```python
from build123d import *

# Parameters (mm, degrees)
SKETCH1_W                 = 31.75
SKETCH1_H                 = 31.75
BOSS_EXTRUDE1_DEPTH       = 5.08
M3_CLEARANCE_HOLE1_D      = 3.4
M3_CLEARANCE_HOLE1_DEPTH  = 15.24
M3_CLEARANCE_HOLE1_TIP    = 1.021463052
SKETCH7_W                 = 31.75
SKETCH7_H                 = 31.75
SKETCH7_R                 = 13.97
BOSS_EXTRUDE2_DEPTH       = 24
M3X0_5_TAPPED_HOLE1_D     = 2.5
M3X0_5_TAPPED_HOLE1_DEPTH = 15.24
M3X0_5_TAPPED_HOLE1_TIP   = 0.751075774
SKETCH12_R                = 4.7625
CUT_EXTRUDE1_DEPTH        = 6.35
CUT_EXTRUDE2_REACH        = 44.849
CUT_EXTRUDE2_END_RADIUS   = 13.97
SKETCH13_W                = 15.618932536
SKETCH13_H                = 11.098734185
CIRPATTERN1_COUNT         = 4
CIRPATTERN2_COUNT         = 4


with BuildPart() as part:
    # Sketch1 → Boss-Extrude1 (new body)
    with BuildSketch(Plane(origin=(0, 0, 0), x_dir=(1, 0, 0), z_dir=(0, 1, 0))):
        Rectangle(SKETCH1_W, SKETCH1_H)
    extrude(amount=BOSS_EXTRUDE1_DEPTH)

    # M3 Clearance Hole1
    with Locations(Plane(origin=(0, 5.08, 0), x_dir=(1, 0, 0), z_dir=(0, 1, 0))):
        with Locations((-5.656854249, 5.656854249), (6.717514421, 6.717514421), (5.656854249, -5.656854249), (-6.717514421, -6.717514421)):
            Hole(M3_CLEARANCE_HOLE1_D / 2, depth=M3_CLEARANCE_HOLE1_DEPTH)
            with Locations((0, 0, -(M3_CLEARANCE_HOLE1_DEPTH + M3_CLEARANCE_HOLE1_TIP / 2))):  # 118° drill point
                Cone(0, M3_CLEARANCE_HOLE1_D / 2, M3_CLEARANCE_HOLE1_TIP, mode=Mode.SUBTRACT)

    # Sketch7 → Boss-Extrude2 (add)
    with BuildSketch(Plane.XZ):
        Rectangle(SKETCH7_W, SKETCH7_H)
        with Locations(Location((0, 0, 0), (0, 0, 270))):
            Circle(SKETCH7_R, mode=Mode.SUBTRACT)
    extrude(amount=BOSS_EXTRUDE2_DEPTH)

    # M3x0.5 Tapped Hole1
    with Locations(Plane(origin=(0, -24, 0), x_dir=(-1, 0, 0), z_dir=(0, -1, 0))):
        with Locations((-12.7, 12.7), (12.7, 12.7), (12.7, -12.7), (-12.7, -12.7)):
            Hole(M3X0_5_TAPPED_HOLE1_D / 2, depth=M3X0_5_TAPPED_HOLE1_DEPTH)
            with Locations((0, 0, -(M3X0_5_TAPPED_HOLE1_DEPTH + M3X0_5_TAPPED_HOLE1_TIP / 2))):  # 118° drill point
                Cone(0, M3X0_5_TAPPED_HOLE1_D / 2, M3X0_5_TAPPED_HOLE1_TIP, mode=Mode.SUBTRACT)

    # Sketch12 → Cut-Extrude1 (cut)
    with BuildSketch(Plane(origin=(0, 0, -15.875), x_dir=(-1, 0, 0), z_dir=(0, 0, -1))):
        with Locations((0, -1.27)):
            Circle(SKETCH12_R)
    cut_extrude1 = extrude(amount=-CUT_EXTRUDE1_DEPTH, mode=Mode.SUBTRACT)

    # Cut-Extrude2: up to this cylinder (the profile starts outside it)
    cut_extrude2_end = Plane(origin=(0, -14.261548, 0), z_dir=(0, 1, 0)) * Cylinder(CUT_EXTRUDE2_END_RADIUS, 118.638, mode=Mode.PRIVATE)
    # Sketch13 → Cut-Extrude2 (cut, up to the surface)
    with BuildSketch(Plane(origin=(0, 0, -15.875), x_dir=(-1, 0, 0), z_dir=(0, 0, -1)), mode=Mode.PRIVATE) as cut_extrude2_sk1:
        with Locations((0, -14.261548471)):
            Rectangle(SKETCH13_W, SKETCH13_H)
    cut_extrude2_tool1 = extrude(cut_extrude2_sk1.sketch, amount=-CUT_EXTRUDE2_REACH, mode=Mode.PRIVATE) - cut_extrude2_end
    cut_extrude2 = cut_extrude2_tool1.solids().sort_by_distance((0, -14.261548, -15.875))[0]
    add(cut_extrude2, mode=Mode.SUBTRACT)

    # CirPattern1: Cut-Extrude2 ×4 about axis
    cirpattern1_axis = Axis((0, 0, 0), (0, 1, 0))
    for i in range(1, CIRPATTERN1_COUNT):
        add(cut_extrude2.rotate(cirpattern1_axis, i * 360 / CIRPATTERN1_COUNT), mode=Mode.SUBTRACT)

    # CirPattern2: Cut-Extrude1 ×4 about axis
    cirpattern2_axis = Axis((0, 0, 0), (0, 1, 0))
    for i in range(1, CIRPATTERN2_COUNT):
        add(cut_extrude1.rotate(cirpattern2_axis, i * 360 / CIRPATTERN2_COUNT), mode=Mode.SUBTRACT)


solid = part.part
```
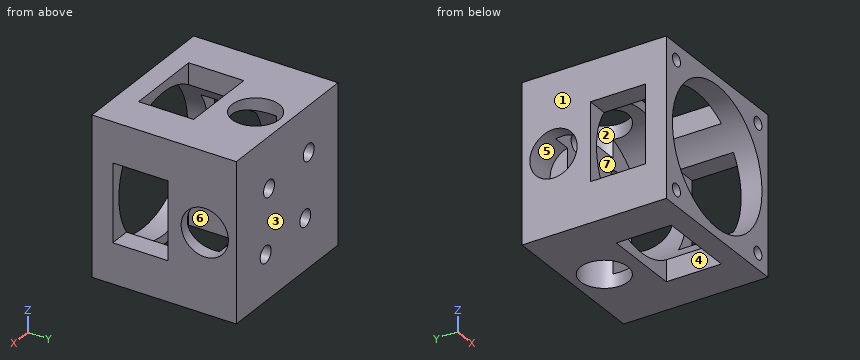
Work out the finished part from the listing and answer in its coordinate system (mm). Face numbers are marked on the shaded views. A direction names the side the tool comes from. Give positions to 0.01 mm unless a question says otherwise; leave off trailing zeros. Loops run counter-clockwise (first coordinate to the right, second up) from the corner with the lowest first, then second, coordinate; pieces in that order, holes last. Notation, with made-up numbers: (76, 37) -> (80, 37) arc R23 ccw to (80, 48) -> close; hole circle Ø11 at (46.5, 4). An arc over 180 degrees is marked (long way). Use CSV: the item, a comma, the result in double quotes.
1. The part is cut by section B-B (x = -1). Write down the section's boundary in (y, z) (3 decimals).
Found:
outline,"(-24, -15.875) -> (-19.811, -15.875) -> (-19.811, -13.934) -> (-24, -13.934) -> close; (-24, 13.934) -> (-19.811, 13.934) -> (-19.811, 15.875) -> (-24, 15.875) -> close; (-8.712, -15.875) -> (-5.926, -15.875) -> (-5.926, -13.934) -> (-8.712, -13.934) -> close; (-8.712, 13.934) -> (-5.926, 13.934) -> (-5.926, 15.875) -> (-8.712, 15.875) -> close; (0, -9.525) -> (3.386, -9.525) -> (3.386, -15.875) -> (5.08, -15.875) -> (5.08, 15.875) -> (3.386, 15.875) -> (3.386, 9.525) -> (0, 9.525) -> close"
2. The part is cut by section A-A (y = -14.5). Write down the section's boundary in (x, z) (3 decimals).
Found:
outline,"(-15.875, -15.875) -> (-7.809, -15.875) -> (-7.809, -11.583) arc R13.97 cw to (-11.583, -7.809) -> (-15.875, -7.809) -> close; (-15.875, 7.809) -> (-11.583, 7.809) arc R13.97 cw to (-7.809, 11.583) -> (-7.809, 15.875) -> (-15.875, 15.875) -> close; (7.809, -15.875) -> (15.875, -15.875) -> (15.875, -7.809) -> (11.583, -7.809) arc R13.97 cw to (7.809, -11.583) -> close; (7.809, 11.583) arc R13.97 cw to (11.583, 7.809) -> (15.875, 7.809) -> (15.875, 15.875) -> (7.809, 15.875) -> close; hole circle Ø2.5 at (-12.7, -12.7); hole circle Ø2.5 at (-12.7, 12.7); hole circle Ø2.5 at (12.7, -12.7); hole circle Ø2.5 at (12.7, 12.7)"
3. A tool of negligible diameter and unlimited length cuts with its end or side. For the marked faces 5, 6 and 7, from which of +Z, -Z, +X, -X, +Y, -Y can it reach the whole face along a straight path? Write none if from no direction.
Found:
face 5,"-X"
face 6,"+Z, -Z"
face 7,"-Y"
4. Straight lines are drawn through the part: line 1 (X direction, y = -17.75, z = -12.7) (3 decimals); line 2 (X direction, y = 1, z = -6.5) (3 decimals). For each, find the intervals that lie inside material, in ascending order.
Found:
line 1,"-15.875 to -13.95, -11.45 to -7.809, 7.809 to 11.45, 13.95 to 15.875"
line 2,"-15.875 to -7.133, -4.181 to 5.031, 8.404 to 15.875"
5. The mould has two halves that part along Y. Classify the marked faces 1, 2, 3 and 4: +Y half, -Y half, draft (parallel to the pull), parting line (faces both ways), or undercut.
Found:
face 1,"draft"
face 2,"undercut"
face 3,"+Y half"
face 4,"undercut"
6. Flat-ended cylindrical pins translate along their axes: pin 1 Ø8 at (x, z) = (-0.5, -4) entering from -Y; pin 2 Ø1.5 at (x, y) = (-3, -1) entering from -Z; pin 3 Ø1.5 at (x, z) = (-12.7, -12.7) entering from -Y; pin 4 Ø1.7 at (x, y) = (0, 1) entering from +Z (3 decimals). Find the tip coordinate at first contact, or state that the pin passes through.
Found:
pin 1,"y = 0"
pin 2,"through"
pin 3,"y = -8.46"
pin 4,"z = 9.525"
7. The part is cut by section D-D (z = -2). Write down the section's boundary in (x, y) (3 decimals), then the cut area to 3 significant figures.
Found:
outline,"(-15.875, -24) -> (-13.826, -24) -> (-13.826, -19.811) -> (-15.875, -19.811) -> close; (-15.875, -8.712) -> (-13.826, -8.712) -> (-13.826, -5.592) -> (-15.875, -5.592) -> close; (-15.875, 3.052) -> (-9.525, 3.052) -> (-9.525, 0) -> (9.525, 0) -> (9.525, 3.052) -> (15.875, 3.052) -> (15.875, 5.08) -> (-15.875, 5.08) -> close; (13.826, -24) -> (15.875, -24) -> (15.875, -19.811) -> (13.826, -19.811) -> close; (13.826, -8.712) -> (15.875, -8.712) -> (15.875, -5.592) -> (13.826, -5.592) -> close"
area,"152 mm^2"
8. The part is cut by section C-C (y = 3). Write down the section's boundary in (x, z) (3 decimals), then the cut area to 3 significant figures.
Found:
outline,"(-15.875, -15.875) -> (-2.109, -15.875) -> (-2.109, -9.525) -> (2.109, -9.525) -> (2.109, -15.875) -> (15.875, -15.875) -> (15.875, -2.109) -> (9.525, -2.109) -> (9.525, 2.109) -> (15.875, 2.109) -> (15.875, 15.875) -> (2.109, 15.875) -> (2.109, 9.525) -> (-2.109, 9.525) -> (-2.109, 15.875) -> (-15.875, 15.875) -> (-15.875, 2.109) -> (-9.525, 2.109) -> (-9.525, -2.109) -> (-15.875, -2.109) -> close; hole circle Ø3.4 at (-6.718, 6.718); hole circle Ø3.4 at (-5.657, -5.657); hole circle Ø3.4 at (5.657, 5.657); hole circle Ø3.4 at (6.718, -6.718)"
area,"865 mm^2"
